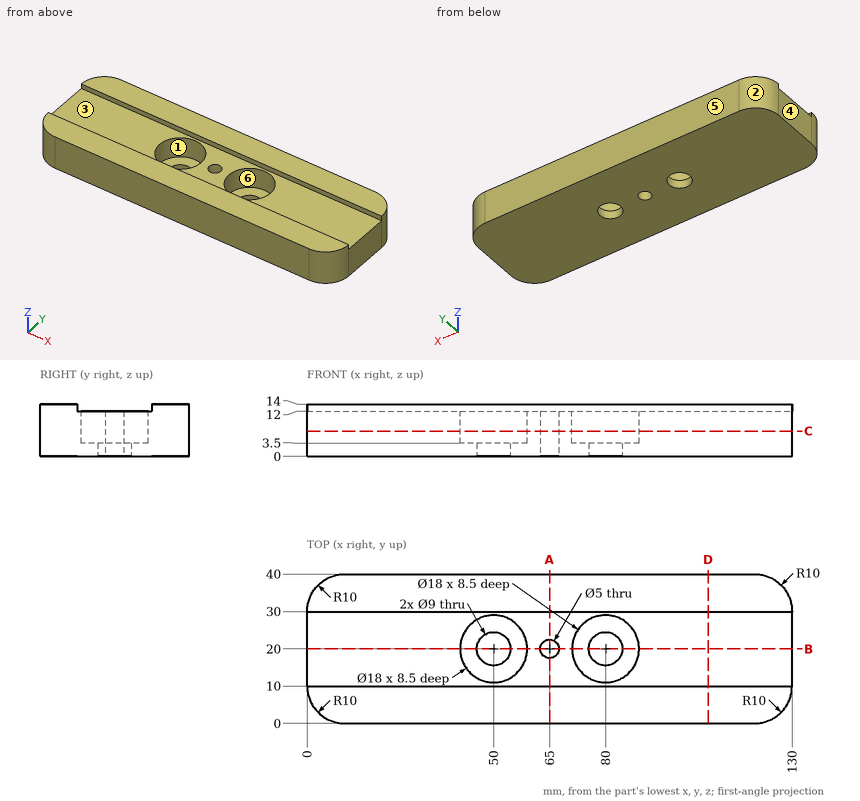
Verification items for this drawing (mm, ordinates from the low corner). A direction names the side the tool comes from. Give positions to 0.01 mm unless a question says otherwise; leave off trailing zeros. Loops run counter-clockwise (first coordinate to the right, second up) from the corner with the lowest first, then second, coordinate; pieces in that order, holes last. Notation, with made-up numbers: M 10,50 L 60,50 A28 ccw 60,79 Z; hole C 84,24 d11. An arc over 180 degrees is marked long. Return JSON: item names as keys, results as strings. Group by question number.
1. Cross-section at B-B on y = 20. Record the boundary of the cut face in (x, z).
2. Cross-section at C-C on z = 6.75. Record the boundary of the cut face in (x, y).
3. Go/stop test with flat-tipped pins: pin 1 (5.5 mm diameter, centred on x = 80, y = 20, fed in from +Z); pin 2 (14.5 mm diameter, centred on x = 52.5, y = 19, fed in from +Z); pin 3 (14.5 mm diameter, centred on x = 50, y = 20, fed in from +Z); pin 4 (5 mm diameter, centred on y = 5, z = 4, fed in from -X). Record where each tip stops, or that it passes through.
4. Tool access check on the marked faces 1, 2 and 3. Record the directions out of +Z, -Z, +X, -X, +Y, -Y that give a thin tool (end or side, any length) a straight path to the whole face; none if there is none.
5. Cross-section at A-A on x = 65. Record the boundary of the cut face in (y, z).
6. Cross-section at D-D on x = 107.5. Record the boundary of the cut face in (y, z), plus the area to 3 significant figures.
7. Thickness scan on L1, parallel to X at y = 21.5, z = 5.25; L2, parallel to Y at x = 50, z = 9.75; L3, parallel to Z at x = 29, y = 25. Record the ranges inside material, lowest first.
8. Mould release check, pull along X, two halves, no side actions. Record for the marked faces 4, 5 and 6: released by +X, released by -X, zero draft, split by the parting line, or undercut.
Return value:
{
 "1": {"outline": "M 0,0 L 45.5,0 L 45.5,3.5 L 41,3.5 L 41,12 L 0,12 Z; M 54.5,0 L 62.5,0 L 62.5,12 L 59,12 L 59,3.5 L 54.5,3.5 Z; M 67.5,0 L 75.5,0 L 75.5,3.5 L 71,3.5 L 71,12 L 67.5,12 Z; M 84.5,0 L 130,0 L 130,12 L 89,12 L 89,3.5 L 84.5,3.5 Z"},
 "2": {"outline": "M 0,10 A10 ccw 10,0 L 120,0 A10 ccw 130,10 L 130,30 A10 ccw 120,40 L 10,40 A10 ccw 0,30 Z; hole C 50,20 d18; hole C 65,20 d5; hole C 80,20 d18"},
 "3": {"pin 1": "through", "pin 2": "z = 12", "pin 3": "z = 3.5", "pin 4": "x = 0.32"},
 "4": {"face 1": "+Z", "face 2": "+Z, -Z, -X, +Y", "face 3": "+Z, +X, -X"},
 "5": {"outline": "M 0,0 L 17.5,0 L 17.5,12 L 10,12 L 10,14 L 0,14 Z; M 22.5,0 L 40,0 L 40,14 L 30,14 L 30,12 L 22.5,12 Z"},
 "6": {"outline": "M 0,0 L 40,0 L 40,14 L 30,14 L 30,12 L 10,12 L 10,14 L 0,14 Z", "area": "520 mm^2"},
 "7": {"L1": "0 to 41.13, 58.87 to 63, 67 to 71.13, 88.87 to 130", "L2": "0 to 11, 29 to 40", "L3": "0 to 12"},
 "8": {"face 4": "released by -X", "face 5": "zero draft", "face 6": "undercut"}
}
